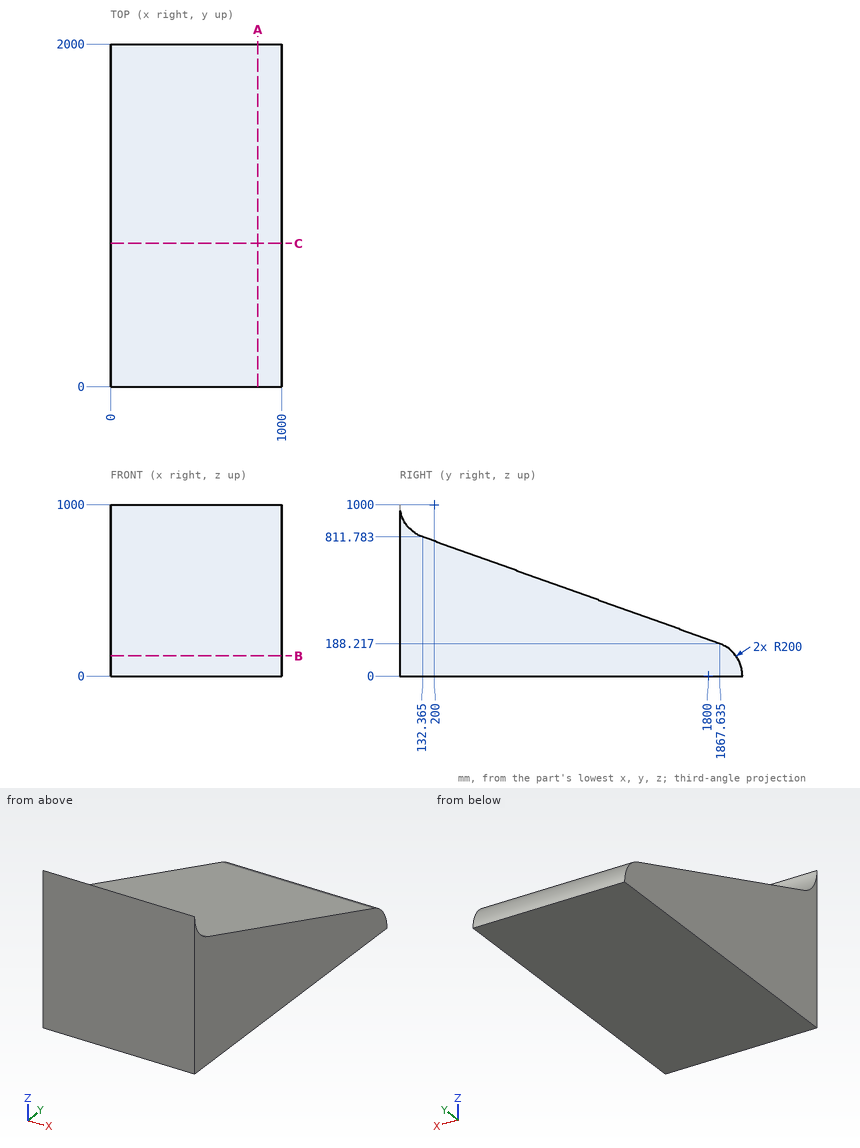
Source: three-view drawing plus pictorial views. Frame: mm from the lowest corner of the part. Round coordinates to 2 decimals unless told otherwise and drop trailing zeros. Order: outer loops, then holes, each group sorted by start corner. A loop starts at its lowest first (then second) coordinate and runs counter-clockwise, first axis right, second up. Notation, with made-up numbers: (-22, 6) -> (20, 6) arc R26 cw to (20, 37) -> close; hole circle Ø5 at (51.5, 21). An arc over 180 degrees is marked (long way). Use one line per item in the form item = value. Start each with the question number.
1. Cut plane C-C (y = 837). Return the cut outline in (x, z).
2. Line query: probe 1 along Z at (x, y) = (468.5, 1115.5) (1 decimal); probe 2 along Y at (x, z) = (282, 949); probe 3 along Y at (x, z) = (377.5, 825) (1 decimal). Output: solid intervals per line, ascending.
3. Cut plane A-A (x = 860). Return the cut outline in (y, z) (1 decimal), then the cut area to 3 significant figures.
4. Pin query (flat end, axial travel): pin 1 Ø3 at (x, y) = (318.5, 1628) entering from +Z. Return the tip coordinate at first contact, or that it passes through.
5. Cut plane B-B (z = 117.5). Return the cut outline in (x, y) (1 decimal).
Solution:
q1.outline = (0, 0) -> (1000, 0) -> (1000, 558.57) -> (0, 558.57) -> close
q2.probe_1 = 0 to 458.5
q2.probe_2 = 0 to 6.61
q2.probe_3 = 0 to 103.2
q3.outline = (0, 0) -> (2000, 0) arc R200 ccw to (1867.6, 188.2) -> (132.4, 811.8) arc R200 cw to (0, 1000) -> close
q3.area = 1,000,000 mm^2
q4.pin_1 = 274.87
q5.outline = (0, 0) -> (1000, 0) -> (1000, 1961.8) -> (0, 1961.8) -> close
